Verification items for the finished model (mm, model axes). Give positions to 0.01 mm unless a question says otherwise; leave off trailing zeros. Write each loop counter-clockwise with the first axis right and the second up, starting at its lowest first coordinate (ties: lowest second). Pieces come first, ordered by that corner, then holes. Notation, with made-up numbers: (69.25, -15) -> (103.25, -15) arc R7 ccw to (103.25, -8) -> close; hole circle Ø7 at (84.25, -8.5). An arc over 180 degrees is marked (long way). Use one line per item in the form item = value. Start each with the question number.
(1) Section check B-B, the plane y = 0.6. Record the cut outline in (x, z), plus the area to 3 significant figures.
(2) Depth check by flat-ended pin: pin 1 Ø3 at (x, z) = (0, 10.5) entering from +Y. Enter the tip coordinate at first touch or a pass-through.
(3) Section check A-A, the plane z = 0. Record the cut outline in (x, y), plus the area to 3 significant figures.
(4) Section check D-D, the plane z = -10.5. Record the cut outline in (x, y).
(5) Scan lines: L1, parallel to X at y = 0.5, z = 3.25; L2, parallel to Z at x = -2.75, y = 0.7; L3, parallel to Z at x = -0.5, y = 1.35. Record each from-to range of solid material in increasing order.
(6) Section check C-C, the plane x = 0. Record the cut outline in (y, z).
from build123d import *

# Parameters (mm, degrees)
CROQUIS1_R              = 13.18
CROQUIS1_R_2            = 5.3
SALIENTE_EXTRUIR1_DEPTH = 2
CROQUIS2_R              = 1.8
CORTAR_EXTRUIR1_DEPTH   = 2
MATRIZC1_COUNT          = 4


with BuildPart() as part:
    # Croquis1 → Saliente-Extruir1 (new body)
    with BuildSketch(Plane(origin=(0, 0, 0), x_dir=(1, 0, 0), z_dir=(0, 1, 0))):
        Circle(CROQUIS1_R)
        Circle(CROQUIS1_R_2, mode=Mode.SUBTRACT)
    extrude(amount=SALIENTE_EXTRUIR1_DEPTH)

    # Croquis2 → Cortar-Extruir1 (cut)
    with BuildSketch(Plane(origin=(0, 2, 0), x_dir=(1, 0, 0), z_dir=(0, 1, 0))):
        with Locations((10.5, 0)):
            Circle(CROQUIS2_R)
    cortar_extruir1 = extrude(amount=-CORTAR_EXTRUIR1_DEPTH, mode=Mode.SUBTRACT)

    # MatrizC1: Cortar-Extruir1 ×4 about axis
    matrizc1_axis = Axis((0, 0, 0), (0, 1, 0))
    for i in range(1, MATRIZC1_COUNT):
        add(cortar_extruir1.rotate(matrizc1_axis, i * 360 / MATRIZC1_COUNT), mode=Mode.SUBTRACT)


solid = part.part
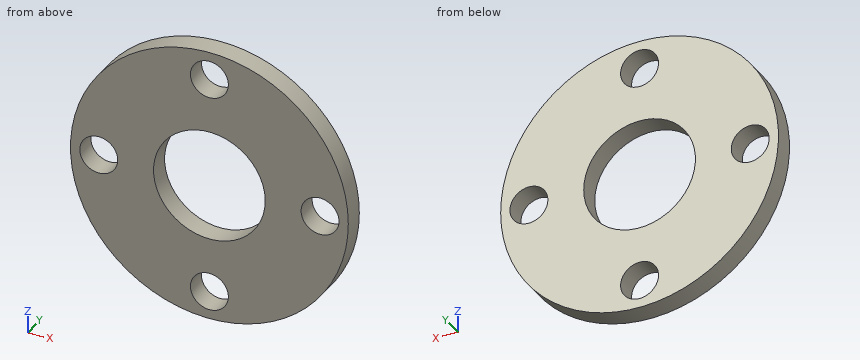
Completed:
q1.outline = circle Ø26.36 at (0, 0); hole circle Ø3.6 at (-10.5, 0); hole circle Ø10.6 at (0, 0); hole circle Ø3.6 at (0, -10.5); hole circle Ø3.6 at (0, 10.5); hole circle Ø3.6 at (10.5, 0)
q1.area = 417 mm²
q2.pin_1 = through
q3.outline = (-13.18, 0) -> (-12.3, 0) -> (-12.3, 2) -> (-13.18, 2) -> close; (-8.7, 0) -> (-5.3, 0) -> (-5.3, 2) -> (-8.7, 2) -> close; (5.3, 0) -> (8.7, 0) -> (8.7, 2) -> (5.3, 2) -> close; (12.3, 0) -> (13.18, 0) -> (13.18, 2) -> (12.3, 2) -> close
q3.area = 17.1 mm²
q4.outline = (-7.97, 0) -> (-1.8, 0) -> (-1.8, 2) -> (-7.97, 2) -> close; (1.8, 0) -> (7.97, 0) -> (7.97, 2) -> (1.8, 2) -> close
q5.L1 = -12.77 to -4.19, 4.19 to 12.77
q5.L2 = -12.89 to -4.53, 4.53 to 12.89
q5.L3 = -13.17 to -12.23, -8.77 to -5.28, 5.28 to 8.77, 12.23 to 13.17
q6.outline = (0, -13.18) -> (2, -13.18) -> (2, -12.3) -> (0, -12.3) -> close; (0, -8.7) -> (2, -8.7) -> (2, -5.3) -> (0, -5.3) -> close; (0, 5.3) -> (2, 5.3) -> (2, 8.7) -> (0, 8.7) -> close; (0, 12.3) -> (2, 12.3) -> (2, 13.18) -> (0, 13.18) -> close
